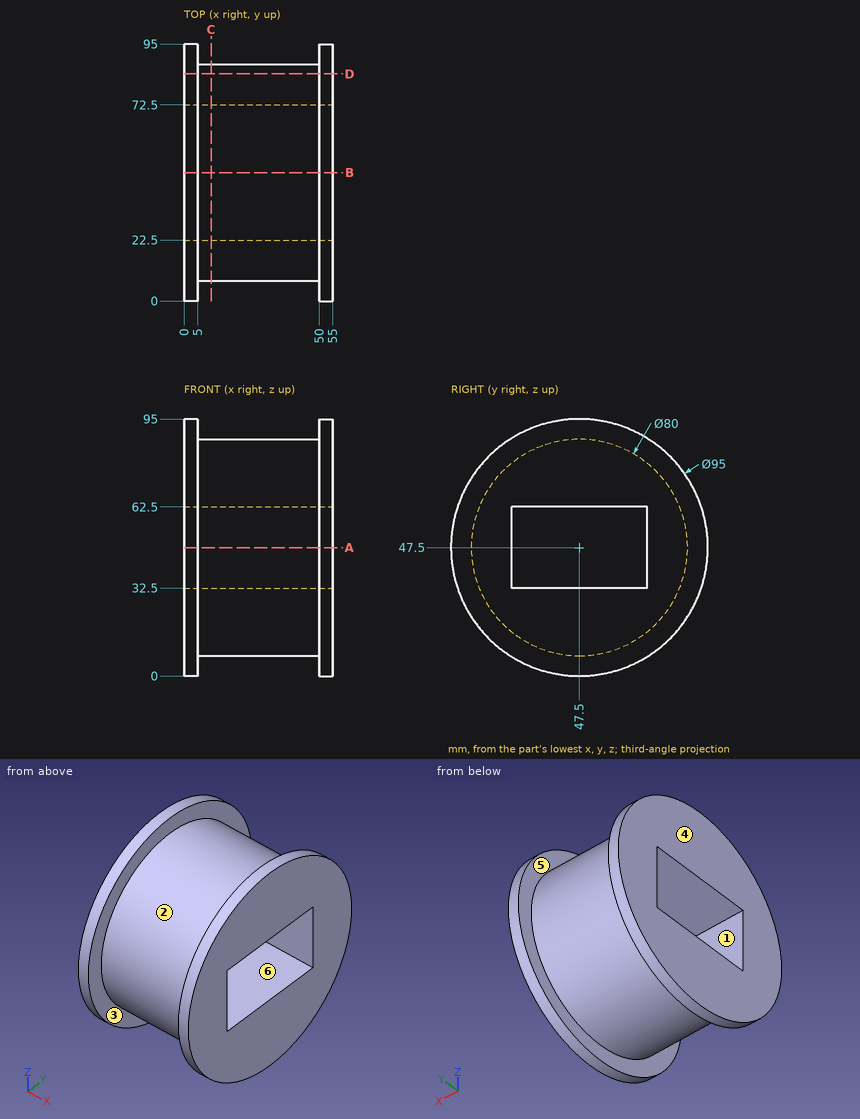
Source: three-view drawing plus pictorial views. Frame: mm from the lowest corner of the part. A direction names the side the tool comes from. Round coordinates to 2 decimals unless told otherwise and drop trailing zeros. Loops run counter-clockwise (first coordinate to the right, second up) from the corner with the lowest first, then second, coordinate; pieces in that order, holes last.
Q1. Section D-D on y = 84. Return loops of the section in (x, z), plus the area to 3 significant figures.
Q2. Access query for the marked faces 4, 5 and 6. Directions: +Z, -Z, +X, -X, +Y, -Y. A direction counts if a zero-diameter tool reaches every point of the face in a straight line with its end or side. Return the directions, or none.
Q3. Pull-direction query (Z, two-part tool) for the marked faces 1, 2 and 3; classes: released by +Z, released by -Z, zero draft, split by the parting line, or undercut.
Q4. Section A-A on z = 47.5. Return loops of the section in (x, y).
Q5. Material intervals for L1, parallel to X at y = 77, z = 81.5; L2, parallel to Y at x = 17, z = 61.5; L3, parallel to Z at x = 37, y = 71, sorted ascending.
Q6. Section C-C on x = 10. Return loops of the section in (y, z), plus the area to 3 significant figures.
Q7. Pin query (flat end, axial travel): P1, Ø25, axis at x = 30.5, y = 43, coming from the -Z side; P2, Ø24, axis at x = 26.5, z = 50, coming from the +Y side; P3, Ø3, axis at x = 25, z = 69, coming from the -Y side. Return the tip coordinate at first contact, or that it passes through.
Q8. Section B-B on y = 47.5. Return loops of the section in (x, z).
Evaluation:
1. outline: (0, 17.1) - (5, 17.1) - (5, 31.14) - (50, 31.14) - (50, 17.1) - (55, 17.1) - (55, 77.9) - (50, 77.9) - (50, 63.86) - (5, 63.86) - (5, 77.9) - (0, 77.9) - close
1. area: 2,080 mm2
2. face 4: +Z, -Z, -X, +Y, -Y
2. face 5: none
2. face 6: +X, -X
3. face 1: undercut
3. face 2: split by the parting line
3. face 3: zero draft
4. outline: (0, 0) - (5, 0) - (5, 7.5) - (50, 7.5) - (50, 0) - (55, 0) - (55, 22.5) - (0, 22.5) - close; (0, 72.5) - (55, 72.5) - (55, 95) - (50, 95) - (50, 87.5) - (5, 87.5) - (5, 95) - (0, 95) - close
5. L1: x = 0 to 5, 50 to 55
5. L2: y = 10.03 to 22.5, 72.5 to 84.97
5. L3: z = 15.13 to 32.5, 62.5 to 79.87
6. outline: circle Ø80 at (47.5, 47.5); hole (22.5, 32.5) - (72.5, 32.5) - (72.5, 62.5) - (22.5, 62.5) - close
6. area: 3,530 mm2
7. P1: stops at z = 7.5
7. P2: stops at y = 87.5
7. P3: stops at y = 12.86
8. outline: (0, 0) - (5, 0) - (5, 7.5) - (50, 7.5) - (50, 0) - (55, 0) - (55, 32.5) - (0, 32.5) - close; (0, 62.5) - (55, 62.5) - (55, 95) - (50, 95) - (50, 87.5) - (5, 87.5) - (5, 95) - (0, 95) - close
